Autodesk Inventor part; units mm, degrees
ref_plane "YZ Plane" through (0, 0, 0) normal (1, 0, 0) x (0, 1, 0)
ref_plane "XZ Plane" through (0, 0, 0) normal (0, 1, 0) x (-1, 0, 0)
ref_plane "XY Plane" through (0, 0, 0) normal (0, 0, 1) x (1, 0, 0)
ref_plane "作業平面1" through (0, 0, 0) normal (0, 0, 1) x (1, 0, 0)
sketch "スケッチ1" plane through (0, 0, 0) normal (0, 0, 1) x (1, 0, 0)
  arc A0 (-6.5014, -6.7164) -> (9.4986, -6.7164) centre (1.4986, -6.7164) ccw
  line L0 (9.4986, -6.7164) -> (9.4986, -0.9651)
  arc A1 (9.4986, -0.9651) -> (9.2306, 0.0349) centre (7.4986, -0.9651) ccw
  line L1 (9.2306, 0.0349) -> (2.6306, 11.4664)
  arc A2 (2.6306, 11.4664) -> (-8.6277, 4.9664) centre (-2.9986, 8.2164) ccw
  line L2 (-8.6277, 4.9664) -> (-6.9034, 1.9797)
  arc A3 (-6.5014, 0.4797) -> (-6.9034, 1.9797) centre (-9.5014, 0.4797) ccw
  line L3 (-6.5014, 0.4797) -> (-6.5014, -6.7164)
  circle A4 centre (-2.9986, 8.2164) radius 3
  circle A5 centre (1.4986, -6.7164) radius 1
  circle A6 centre (5.9986, -6.7164) radius 0.9
  line L4 (5.9986, -6.7164) -> (1.4986, -6.7164) construction
  circle A7 centre (3.7486, -2.8193) radius 0.9
  circle A8 centre (-0.7514, -2.8193) radius 0.9
  circle A9 centre (-3.0014, -6.7164) radius 0.9
  circle A10 centre (-0.7514, -10.6135) radius 0.9
  circle A11 centre (3.7486, -10.6135) radius 0.9
  circle A12 centre (1.4986, -6.7164) radius 3
  arc A13 (-6.5014, 2.1559) -> (3.9296, 9.2164) centre (-2.9986, 8.2164) ccw
  circle A14 centre (1.4986, -6.7164) radius 1
  line L5 (-6.5014, 2.1559) -> (-6.5014, 0.4797)
  circle A15 centre (3.9986, -11.0465) radius 1.25
  point P0 (0, 0)
  dimension "d0" = 4.5
  dimension "d1" = 1.8
  dimension "d4" = 360
  dimension "d6" = 6
  dimension "d7" = 7
  dimension "d10" = 2
extrude "押し出し1" add sketch "スケッチ1" along normal blind 2 contours L3 L5 A13 L1 A1 L0 A0 | A11 A15 | A12 picked at (4.4817, -11.8763)
sketch "スケッチ2" plane through (0, 0, 2) normal (0, 0, 1) x (1, 0, 0)
  line L0 (9.2306, 0.0349) -> (3.9296, 9.2164)
  line L1 (-6.5014, 2.1559) -> (-6.5014, -6.7164)
  arc A0 (-6.5014, -6.7164) -> (9.4986, -6.7164) centre (1.4986, -6.7164) ccw
  line L2 (9.4986, -6.7164) -> (9.4986, -0.9651)
  arc A1 (9.4986, -0.9651) -> (9.2306, 0.0349) centre (7.4986, -0.9651) ccw
  circle A2 centre (3.7486, -10.6135) radius 0.9
  circle A3 centre (-0.7514, -10.6135) radius 0.9
  circle A4 centre (-3.0014, -6.7164) radius 0.9
  circle A5 centre (-0.7514, -2.8193) radius 0.9
  circle A6 centre (3.7486, -2.8193) radius 0.9
  circle A7 centre (5.9986, -6.7164) radius 0.9
  circle A8 centre (1.4986, -6.7164) radius 1
  circle A9 centre (1.4986, -6.7164) radius 3
  arc A10 (-6.5014, 2.1559) -> (3.9296, 9.2164) centre (-2.9986, 8.2164) ccw
  point P0 (0, 0)
  dimension "d11" = 6
extrude "押し出し2" cut sketch "スケッチ2" against normal blind 1.15 contours A9
fillet "フィレット1" radius 2 2 edges at (3.9296, 9.2164, 1) (-6.5014, 2.1559, 1)
properties part number "Motor_Mount"
Build history of the part. All positions in model axes, mm. Round coordinates to 2 decimals unless told otherwise and drop trailing zeros. Write each loop counter-clockwise with the first axis right and the second up, starting at its lowest first coordinate (ties: lowest second). Pieces come first, ordered by that corner, then holes. Notation, with made-up numbers: M 3.5,58 L 19.5,58 A30 cw 19.5,83 Z; hole C 40.5,44.25 d11. An arc over 180 degrees is marked long. Answer as a JSON object with one key per item and string values. Group by question number.
(1) Cut at B-B (y = -6.5). Give the cut face in (x, z) (3 decimals).
(2) Cut at A-A (x = 1.5). Give the cut face in (y, z), and give its area (3 significant figures).
(3) Cut at C-C (z = 1.7). Give the cut face in (x, y), and give its area (3 significant figures).
(4) Drill centre lines: L1, parallel to X at y = -2.75, z = 0.75; L2, parallel to X at y = -3.5, z = 1.6; L3, parallel to X at y = -7, z = 1.8. Where is each one in solid material? Low to high.
(5) Mould opens along X. For faces 1 (the cylindrical face through (-3.716, -6.169, 0.986)), 2 (the flat face through (1, -4, 0)), 3 (the flat face through (7.9, 2.34, 0.99)), 4 (the flat face through (3, -7, 0.85)) say: pulls with the +X half, pulls with the -X half, needs draft (parallel to the pull), parting line crosses it, or undercut.
(6) Cut at D-D (y = -9.5). Give the cut face in (x, z).
(7) Flat gauge pins, fed straight in: pin 1 (1 mm diameter, centred on y = 1.5, z = 0.5, fed in from +X); pin 2 (1.1 mm diameter, centred on x = -0.75, y = -2.82, fed in from -Z); pin 3 (1.8 mm diameter, centred on x = 0, y = -6.5, fed in from +Z). Where does each tip first touch, or does it go through?
Responses:
{
 "1": {"outline": "M -6.501,0 L -3.875,0 L -3.875,2 L -6.501,2 Z; M -2.128,0 L 0.522,0 L 0.522,0.85 L -1.494,0.85 L -1.494,2 L -2.128,2 Z; M 2.475,0 L 5.125,0 L 5.125,2 L 4.491,2 L 4.491,0.85 L 2.475,0.85 Z; M 6.872,0 L 9.499,0 L 9.499,2 L 6.872,2 Z"},
 "2": {"outline": "M -14.72,0 L -7.72,0 L -7.72,0.85 L -9.72,0.85 L -9.72,2 L -14.72,2 Z; M -5.72,0 L 2.85,0 L 2.85,2 L -3.72,2 L -3.72,0.85 L -5.72,0.85 Z", "area": "26.5 mm2"},
 "3": {"outline": "M -6.5,-6.72 A8 ccw 9.5,-6.72 L 9.5,-0.97 A2 ccw 9.23,0.03 L 6.53,4.72 A2 ccw 3.06,4.72 A7 cw -4.17,1.31 A2 ccw -6.5,-0.66 Z; hole C -3,-6.72 d1.8; hole C -0.75,-10.61 d1.8; hole C -0.75,-2.82 d1.8; hole C 1.5,-6.72 d6; hole C 3.75,-10.61 d1.8; hole C 3.75,-2.82 d1.8; hole C 6,-6.72 d1.8", "area": "207 mm2"},
 "4": {"L1": "x = -6.5 to -1.65, 0.15 to 2.85, 4.65 to 9.5", "L2": "x = -6.5 to -1.34, -0.16 to 3.16, 4.34 to 9.5", "L3": "x = -6.5 to -3.86, -2.15 to -1.49, 4.49 to 5.14, 6.85 to 9.49"},
 "5": {"face 1": "undercut", "face 2": "needs draft", "face 3": "pulls with the +X half", "face 4": "undercut"},
 "6": {"outline": "M -6,0 L 9,0 L 9,2 L 2.62,2 L 2.62,0.85 L 0.38,0.85 L 0.38,2 L -6,2 Z"},
 "7": {"pin 1": "stops at x = 8.67", "pin 2": "passes through", "pin 3": "stops at z = 0.85"}
}
